Verification items for the finished model (mm, model axes). A direction names the side the tool comes from. Give positions to 0.01 mm unless a question says otherwise; leave off trailing zeros. Order: outer loops, then holes, each group sorted by start corner. A loop starts at its lowest first (then second) coordinate and runs counter-clockwise, first axis right, second up.
(1) Access from +Z, -Z, +X, -X, +Y, -Y to the whole of each face (thin tool, end or side, straight path). Record for faces 1 (the face through (-21.633, 12.53, 0.035)), 2 (the face through (-0.54, -12.32, -2.44)).
(2) Sectioned sample at B-B on z = 57. Record the cut outline in (x, y), plus the area to 3 significant figures.
(3) Gauge pin test, flat ends, axial feed: pin 1 (10 mm diameter, centred on x = 10.5, z = 85, fed in from +Y); pin 2 (6 mm diameter, centred on x = -3.5, z = 30.5, fed in from +Y); pin 3 (4 mm diameter, centred on x = 8, y = 8, fed in from -Z); pin 4 (1.5 mm diameter, centred on x = -0.5, z = 106, fed in from +Y). Record the tip position at first contact, or that the pin passes through.
(4) Mould release check, pull along X, two halves, no side actions. Record for faces 3 (the face through (0, 0, 125)), 4 (the face through (10.94, 5.69, -2.44)), 5 (the face through (2.385, 0.751, 62.259)), 6 (the face through (-10.4, 6.63, -2.44)): pulls with the +X half, pulls with the -X half, needs draft (parallel to the pull), parting line crosses it, or undercut.
(5) Sectioned sample at A-A on z = 0. Record the cut outline in (x, y).
(6) Scan lines: L1, parallel to Z at x = -6, y = 2.5; L2, parallel to X at y = -0.5, z = 63; L3, parallel to Y at x = 1.5, z = 78.5. Record each from-to range of solid material in increasing order.
```python
from build123d import *

# Parameters (mm, degrees)
F0_R     = 2.5
F1_DEPTH = 25
F3_COUNT = 3
F2_R     = 2.5
F4_DEPTH = 125


with BuildPart() as f1:
    # F0 (on Front) → F1 (new body)
    with BuildSketch(Plane.XZ):
        Circle(F0_R)
    extrude(amount=F1_DEPTH)


with BuildPart() as f3_1:
    # F3: instance of F1
    add(f1.part.rotate(Axis((0, 0, 0), (0, 0, 1)), 1 * 360 / F3_COUNT))


with BuildPart() as f3_2:
    # F3: instance of F1
    add(f1.part.rotate(Axis((0, 0, 0), (0, 0, 1)), 2 * 360 / F3_COUNT))


with BuildPart() as f1_1:
    add(f1.part)

    add(f3_1.part)  # F4 merges F3_1

    add(f3_2.part)  # F4 merges F3_2
    # F2 (on Top) → F4 (join)
    with BuildSketch(Plane.XY):
        Circle(F2_R)
    extrude(amount=F4_DEPTH)


solid = f1_1.part
```
Ans:
1. face 1: +Z, -Z, -X, +Y
1. face 2: -Y
2. outline: circle Ø5 at (0, 0)
2. area: 19.6 mm2
3. pin 1: passes through
3. pin 2: stops at y = 2.45
3. pin 3: stops at z = -2.32
3. pin 4: stops at y = 2.5
4. face 3: needs draft
4. face 4: undercut
4. face 5: parting line crosses it
4. face 6: undercut
5. outline: (-22.9, 10.33) - (-2.5, -1.44) - (-2.5, -25) - (2.5, -25) - (2.5, -1.44) - (22.9, 10.33) - (20.4, 14.67) - (0, 2.89) - (-20.4, 14.67) - close
6. L1: z = -2.36 to 2.36
6. L2: x = -2.45 to 2.45
6. L3: y = -2 to 2
